Design review of the part built by this model. Coordinates are the model's own, in mm. Coordinates: 2 decimals unless noted, no trailing zeros. Loops run counter-clockwise (first coordinate to the right, second up) from the corner with the lowest first, then second, coordinate; pieces in that order, holes last. Notation, with made-up numbers: (2, -29.75) -> (49, -29.75) arc R3 ccw to (49, -25.75) -> close; hole circle Ø1 at (55, -4.75). An arc over 180 degrees is marked (long way). One line per item, written item: value. Start each with the question number.
1. Add section B-B on z = -1.75. Write out the cut boundary in (x, y).
2. Add section A-A on x = 0. Write out the cut boundary in (y, z), plus the area to 3 significant figures.
3. For probe 1 along Z at (x, y) = (-0.1, -0.1); probe 2 along Y at (x, z) = (0.05, 2.75); probe 3 along X at (y, z) = (0.1, 2.5), list the stretches that pass through material, from the lowest coordinate up.
```python
from build123d import *

# Parameters (mm, degrees)
SKETCH_1_R           = 0.1016
EXTRUDE_1_DEPTH      = 4
EXTRUDE_2_DEPTH      = 3.9
EXTRUDE_2_DEPTH_BACK = 3
SKETCH_2_R           = 0.19


with BuildPart() as part:
    # 草图1 → 凸台-拉伸1 (new, symmetric)
    with BuildSketch(Plane.XY):
        Circle(SKETCH_1_R)
    extrude(amount=EXTRUDE_1_DEPTH, both=True)

    # 草图2 → 凸台-拉伸2 (add, two sides: drawn at the far end of the back side and taken through both)
    with BuildSketch(Plane.XY.offset(-EXTRUDE_2_DEPTH_BACK)):
        with Locations((0, 0.001129958)):
            Circle(SKETCH_2_R)
    extrude(amount=EXTRUDE_2_DEPTH + EXTRUDE_2_DEPTH_BACK)


solid = part.part
```
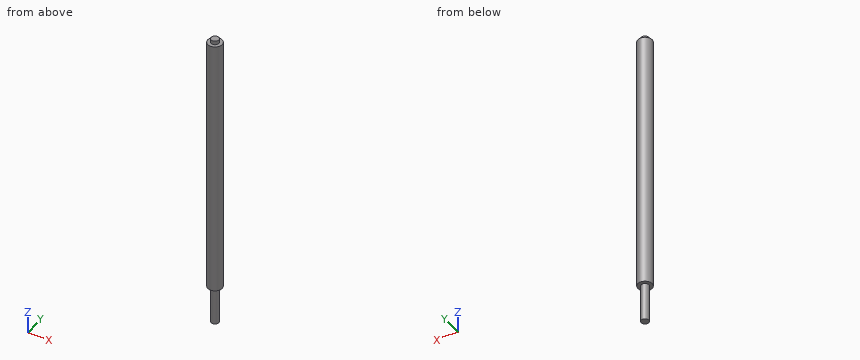
Worked answers:
1. outline: circle Ø0.38 at (0, 0)
2. outline: (-0.19, -3) -> (-0.1, -3) -> (-0.1, -4) -> (0.1, -4) -> (0.1, -3) -> (0.19, -3) -> (0.19, 3.9) -> (0.1, 3.9) -> (0.1, 4) -> (-0.1, 4) -> (-0.1, 3.9) -> (-0.19, 3.9) -> close
2. area: 2.85 mm²
3. probe 1: z = -3 to 3.9
3. probe 2: y = -0.18 to 0.18
3. probe 3: x = -0.16 to 0.16
